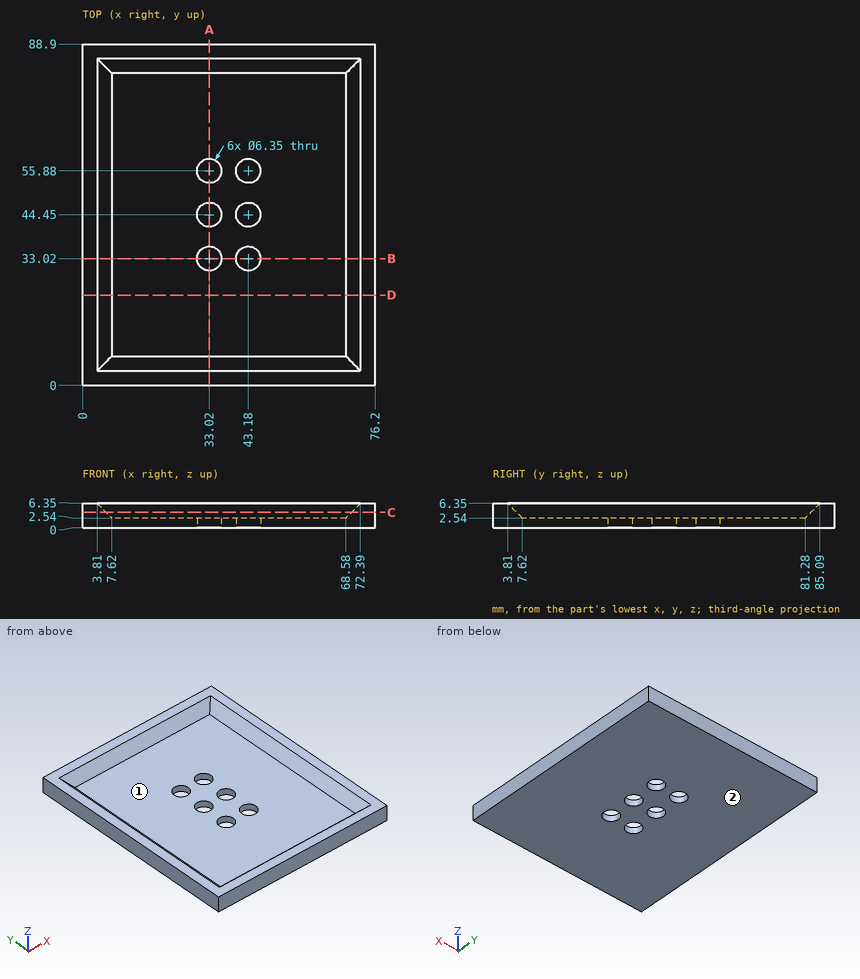
Verification items for this drawing (mm, ordinates from the low corner). Coordinates: 2 decimals unless noted, no trailing zeros. Write each loop counter-clockwise with the first axis right and the second up, starting at its lowest first coordinate (ties: lowest second). Pieces come first, ordered by that corner, then holes. Notation, with made-up numbers: M 58,17 L 90,17 A20 cw 90,35 Z; hole C -11,37 d5. An arc over 180 degrees is marked long. Use one line per item in the form item = value. Start each with the question number.
1) Section check B-B on y = 33.02. Enter the section's corners in (x, z) (3 decimals), and give its area (3 significant figures).
2) Section check D-D on y = 23.5. Enter the section's corners in (x, z).
3) Go/stop test with flat-tipped pins: pin 1 Ø12 at (x, y) = (41.5, 61) entering from +Z; pin 2 Ø5 at (x, y) = (43.18, 44.45) entering from +Z. Record where each tip stops, or that it passes through.
4) Section check C-C on z = 4. Enter the section's corners in (x, y), and give its area (3 significant figures).
5) Release check for a two-part mould opening along X. For the marked faces 1 and 2 record: pulls with the +X half, pulls with the -X half, needs draft (parallel to the pull), parting line crosses it, or undercut.
6) Thickness scan on probe 1 along Y at (x, z) = (43.18, 1.5) (3 decimals); probe 2 along Y at (x, z) = (40.5, 2); probe 3 along Z at (x, y) = (30, 62). Record the ranges inside material, lowest first. Write a range as from..to.
7) Section check A-A on x = 33.02. Enter the section's corners in (y, z) (3 decimals), and give its area (3 significant figures).
Responses:
q1.outline = M 0,0 L 29.845,0 L 29.845,2.54 L 7.62,2.54 L 3.81,6.35 L 0,6.35 Z; M 36.195,0 L 40.005,0 L 40.005,2.54 L 36.195,2.54 Z; M 46.355,0 L 76.2,0 L 76.2,6.35 L 72.39,6.35 L 68.58,2.54 L 46.355,2.54 Z
q1.area = 205 mm2
q2.outline = M 0,0 L 76.2,0 L 76.2,6.35 L 72.39,6.35 L 68.58,2.54 L 7.62,2.54 L 3.81,6.35 L 0,6.35 Z
q3.pin_1 = 2.54
q3.pin_2 = through
q4.outline = M 0,0 L 76.2,0 L 76.2,88.9 L 0,88.9 Z; hole M 6.16,6.16 L 70.04,6.16 L 70.04,82.74 L 6.16,82.74 Z
q4.area = 1,880 mm2
q5.face_1 = undercut
q5.face_2 = needs draft
q6.probe_1 = 0..29.845, 36.195..41.275, 47.625..52.705, 59.055..88.9
q6.probe_2 = 0..31.32, 34.72..42.75, 46.15..54.18, 57.58..88.9
q6.probe_3 = 0..2.54
q7.outline = M 0,0 L 29.845,0 L 29.845,2.54 L 7.62,2.54 L 3.81,6.35 L 0,6.35 Z; M 36.195,0 L 41.275,0 L 41.275,2.54 L 36.195,2.54 Z; M 47.625,0 L 52.705,0 L 52.705,2.54 L 47.625,2.54 Z; M 59.055,0 L 88.9,0 L 88.9,6.35 L 85.09,6.35 L 81.28,2.54 L 59.055,2.54 Z
q7.area = 221 mm2
